Work out the finished part from the listing and answer in its coordinate system (mm). Round coordinates to 2 decimals unless told otherwise and drop trailing zeros. Loops run counter-clockwise (first coordinate to the right, second up) from the corner with the lowest first, then second, coordinate; pieces in that order, holes last. Notation, with made-up numbers: (38.5, 4.25) -> (81.5, 4.25) arc R12 cw to (81.5, 27.25) -> close; hole circle Ø1 at (29, -9.5). An arc over 180 degrees is marked (long way). Write item = value, one per line. Start each with the question number.
```python
from build123d import *

# Parameters (mm, degrees)
F0_R     = 22.425
F1_DEPTH = 49
F2_R     = 0.4
F3_DEPTH = 31


with BuildPart() as f1:
    # F0 (on Front) → F1 (new body)
    with BuildSketch(Plane.XZ):
        Circle(F0_R)
    extrude(amount=F1_DEPTH)

    # F2 (on Top) → F3 (cut)
    with BuildSketch(Plane.XY):
        with Locations((0, -1.5)):
            Circle(F2_R)
        with Locations((0, -3)):
            Circle(F2_R)
        with Locations((0, -4.5)):
            Circle(F2_R)
        with Locations((0, -6)):
            Circle(F2_R)
        with Locations((0, -7.5)):
            Circle(F2_R)
        with Locations((0, -9)):
            Circle(F2_R)
        with Locations((0, -10.5)):
            Circle(F2_R)
        with Locations((0, -12)):
            Circle(F2_R)
        with Locations((0, -13.5)):
            Circle(F2_R)
        with Locations((0, -15)):
            Circle(F2_R)
        with Locations((0, -16.5)):
            Circle(F2_R)
        with Locations((0, -18)):
            Circle(F2_R)
        with Locations((0, -19.5)):
            Circle(F2_R)
        with Locations((0, -21)):
            Circle(F2_R)
        with Locations((0, -22.5)):
            Circle(F2_R)
        with Locations((0, -24)):
            Circle(F2_R)
        with Locations((0, -25.5)):
            Circle(F2_R)
        with Locations((0, -27)):
            Circle(F2_R)
        with Locations((0, -28.5)):
            Circle(F2_R)
        with Locations((0, -30)):
            Circle(F2_R)
        with Locations((0, -31.5)):
            Circle(F2_R)
        with Locations((0, -33)):
            Circle(F2_R)
        with Locations((0, -34.5)):
            Circle(F2_R)
        with Locations((0, -36)):
            Circle(F2_R)
        with Locations((0, -37.5)):
            Circle(F2_R)
        with Locations((0, -39)):
            Circle(F2_R)
        with Locations((0, -40.5)):
            Circle(F2_R)
        with Locations((0, -42)):
            Circle(F2_R)
        with Locations((0, -43.5)):
            Circle(F2_R)
        with Locations((0, -45)):
            Circle(F2_R)
        with Locations((0, -46.5)):
            Circle(F2_R)
        with Locations((0, -48)):
            Circle(F2_R)
    extrude(amount=F3_DEPTH, mode=Mode.SUBTRACT)


solid = f1.part
```
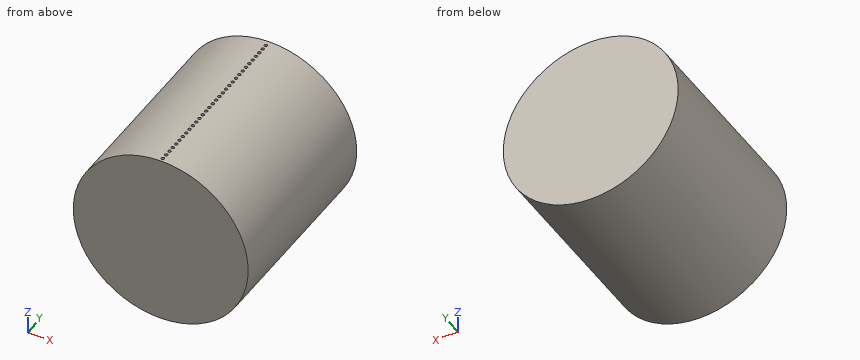
Item 1: Section A-A (z = -10) is taken. Determine the outline of the cut face in (x, y), then the cut area to 3 significant figures.
Item 2: Flat-ended cylindrical pins translate along their axes: pin 1 (10 mm diameter, centred on x = -9, z = 14.5, fed in from +Y); pin 2 (0.6 mm diameter, centred on x = 0, y = -16.5, fed in from +Z); pin 3 (1 mm diameter, centred on x = 13.5, y = -25.5, fed in from +Z); pin 4 (1.5 mm diameter, centred on y = -44, z = 5.5, fed in from +X). Find the tip coordinate at first contact, or state that the pin passes through.
Item 3: Section B-B (x = -16) is taken. Determine the outline of the cut face in (y, z), then the cut area to 3 significant figures.
Item 4: Find the intervals of material crossed by line 1 along X through (y, z) = (-39, 19.5); line 2 along X through (y, z) = (-28.5, 11.75); line 3 along X through (y, z) = (-4, -6.5), in increasing order. Write a range as [from, to].
Worked answers:
q1.outline = (-20.07, -49) -> (20.07, -49) -> (20.07, 0) -> (-20.07, 0) -> close
q1.area = 1,970 mm2
q2.pin_1 = 0
q2.pin_2 = 0
q2.pin_3 = 18.27
q2.pin_4 = 21.92
q3.outline = (-49, -15.71) -> (0, -15.71) -> (0, 15.71) -> (-49, 15.71) -> close
q3.area = 1,540 mm2
q4.line_1 = [-11.07, -0.4], [0.4, 11.07]
q4.line_2 = [-19.1, -0.4], [0.4, 19.1]
q4.line_3 = [-21.46, 21.46]
